Geometry: final body of the model. Coordinates: model frame, mm. Face numbers are marked on the shaded views. Coordinates: 2 decimals unless noted, no trailing zeros. Order: outer loops, then holes, each group sorted by start corner. A loop starts at its lowest first (then second) coordinate and runs counter-clockwise, first axis right, second up. Notation, with made-up numbers: (-7.5, 54) - (44.5, 54) arc R27 cw to (44.5, 79) - close; hole circle Ø8 at (-9, 80). An arc over 180 degrees is marked (long way). Use one line per item in the form item = value. Start each with the question number.
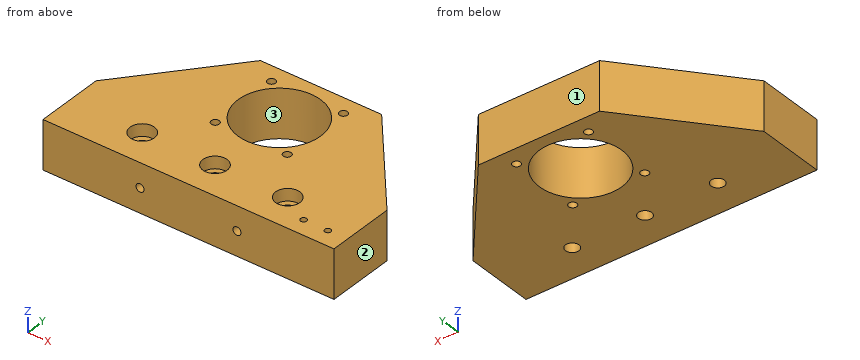
```python
from build123d import *

# Parameters (mm, degrees)
BOSS_EXTRUDE1_DEPTH            = 20
CBORE_FOR_M5_SHCS1_D           = 5.5
CBORE_FOR_M5_SHCS1_CBORE_D     = 10
CBORE_FOR_M5_SHCS1_CBORE_DEPTH = 5
SKETCH4_R                      = 17
CUT_EXTRUDE1_DEPTH             = 95.339811321
M4_TAPPED_HOLE1_D              = 3.3
M4_TAPPED_HOLE2_D              = 3.3
M4_TAPPED_HOLE2_DEPTH          = 15
M4_TAPPED_HOLE2_TIP            = 0.991420021
M3_TAPPED_HOLE1_D              = 2.5
M3_TAPPED_HOLE1_DEPTH          = 7.5
M3_TAPPED_HOLE1_TIP            = 0.751075774


with BuildPart() as part:
    # Sketch1 → Boss-Extrude1 (new body)
    with BuildSketch(Plane.XY):
        Polygon((60, 0), (-60, 0), (-60, 28), (-25, 70), (25, 70), (60, 28), align=None)
    extrude(amount=BOSS_EXTRUDE1_DEPTH)

    # CBORE for M5 SHCS1 (through all)
    with Locations(Plane(origin=(-30, 14, 20), x_dir=(1, 0, 0), z_dir=(0, 0, 1))):
        with Locations((0, 0), (30, 0), (60, 0)):
            CounterBoreHole(CBORE_FOR_M5_SHCS1_D / 2, CBORE_FOR_M5_SHCS1_CBORE_D / 2, CBORE_FOR_M5_SHCS1_CBORE_DEPTH)

    # Sketch4 → Cut-Extrude1 (cut, through all)
    with BuildSketch(Plane.XY.offset(20)):
        with Locations((0, 48)):
            Circle(SKETCH4_R)
    extrude(amount=-CUT_EXTRUDE1_DEPTH, mode=Mode.SUBTRACT)

    # M4 Tapped Hole1 (through all)
    with Locations(Plane(origin=(-14.849242405, 62.849242405, 20), x_dir=(1, 0, 0), z_dir=(0, 0, 1))):
        with Locations((0, 0), (29.69848481, 0), (29.69848481, -29.69848481), (0, -29.69848481)):
            Hole(M4_TAPPED_HOLE1_D / 2)

    # M4 Tapped Hole2
    with Locations(Plane(origin=(0, 0, 0), x_dir=(-1, 0, 0), z_dir=(0, -1, 0))):
        with Locations((20, -10), (-20, -10)):
            Hole(M4_TAPPED_HOLE2_D / 2, depth=M4_TAPPED_HOLE2_DEPTH)
            with Locations((0, 0, -(M4_TAPPED_HOLE2_DEPTH + M4_TAPPED_HOLE2_TIP / 2))):  # 118° drill point
                Cone(0, M4_TAPPED_HOLE2_D / 2, M4_TAPPED_HOLE2_TIP, mode=Mode.SUBTRACT)

    # M3 Tapped Hole1
    with Locations(Plane(origin=(42, 7, 20), x_dir=(1, 0, 0), z_dir=(0, 0, 1))):
        with Locations((0, 0), (10, 0)):
            Hole(M3_TAPPED_HOLE1_D / 2, depth=M3_TAPPED_HOLE1_DEPTH)
            with Locations((0, 0, -(M3_TAPPED_HOLE1_DEPTH + M3_TAPPED_HOLE1_TIP / 2))):  # 118° drill point
                Cone(0, M3_TAPPED_HOLE1_D / 2, M3_TAPPED_HOLE1_TIP, mode=Mode.SUBTRACT)


solid = part.part
```
(1) Draft query along X for the marked faces 1, 2 and 3. Return one class per face: released by +X, released by -X, zero draft, split by the parting line, or undercut.
(2) Cut plane C-C on y = 55.5. Return the cut outline in (x, z), plus the area to 3 significant figures.
(3) Material intervals for L1, parallel to Y at x = 0, z = 9.25; L2, parallel to Z at x = -20, y = 7; L3, parallel to X at y = 7, z = 15.75, sorted ascending. Write a range as from..to.
(4) Cut plane D-D on z = 5. Count the separate pieces of the cut face and the enclosed holes in it, plus the area to 3 significant figures.
(5) Cut plane B-B on x = -30. Return the cut outline in (y, z), plus the area to 3 significant figures.
(6) Contact query for flat-ended pins moving along their axis: pin 1 Ø10 at (y, z) = (45, 9) entering from -X; pin 2 Ø8 at (x, z) = (43.5, 14.5) entering from +Y; pin 3 Ø9 at (x, y) = (30, 14) entering from +Z. Output: stop coordinate, or through.
(7) Cut plane A-A on x = 0. Return the cut outline in (y, z).
Check sheet entries:
q1.face_1 = zero draft
q1.face_2 = released by +X
q1.face_3 = undercut
q2.outline = (-37.08, 0) - (-15.26, 0) - (-15.26, 20) - (-37.08, 20) - close; (15.26, 0) - (37.08, 0) - (37.08, 20) - (15.26, 20) - close
q2.area = 873 mm^2
q3.L1 = 0..11.25, 16.75..31, 65..70
q3.L2 = 0..8.35, 11.65..20
q3.L3 = -60..40.75, 43.25..50.75, 53.25..60
q4.separate_pieces = 1
q4.enclosed_holes = 8
q4.area = 5,920 mm^2
q5.outline = (0, 0) - (11.25, 0) - (11.25, 15) - (9, 15) - (9, 20) - (0, 20) - close; (16.75, 0) - (64, 0) - (64, 20) - (19, 20) - (19, 15) - (16.75, 15) - close
q5.area = 1,150 mm^2
q6.pin_1 = -50
q6.pin_2 = 52.6
q6.pin_3 = 15
q7.outline = (0, 0) - (11.25, 0) - (11.25, 15) - (9, 15) - (9, 20) - (0, 20) - close; (16.75, 0) - (31, 0) - (31, 20) - (19, 20) - (19, 15) - (16.75, 15) - close; (65, 0) - (70, 0) - (70, 20) - (65, 20) - close
